```python
from build123d import *

# Parameters (mm, degrees)
SKETCH2_W           = 2.25
SKETCH2_H           = 25
BOSS_EXTRUDE1_DEPTH = 4
SKETCH4_OUTSIDE_W   = 76.3
SKETCH4_OUTSIDE_H   = 75.213
SKETCH4_OUTSIDE_R   = 3.514702834
CUT_EXTRUDE1_DEPTH  = 30
CUT_EXTRUDE1_TAPER  = 45


with BuildPart() as part:
    # Sketch2 → Revolve1 (revolve)
    with BuildSketch(Plane.XY):
        with Locations((1.125, 12.5)):
            Rectangle(SKETCH2_W, SKETCH2_H)
    revolve(axis=Axis((2.25, 25, 0), (0, -1, 0)))

    # Sketch3 → Boss-Extrude1 (add)
    with BuildSketch(Plane.XZ):
        Polygon((6.308429255, 0.02726243), (4.279214628, 3.541965265), (0.220785372, 3.541965265), (-1.808429255, 0.02726243), (0.220785372, -3.487440404), (4.279214628, -3.487440404), align=None)
    extrude(amount=BOSS_EXTRUDE1_DEPTH)

    # Sketch4 outside → Cut-Extrude1 (cut, through all)
    with BuildSketch(Plane(origin=(0, -4, 0), x_dir=(-1, 0, 0), z_dir=(0, -1, 0))):
        with Locations((-2.25, -0.0275)):
            Rectangle(SKETCH4_OUTSIDE_W, SKETCH4_OUTSIDE_H)
        with Locations((-2.25, -0.02726243)):
            Circle(SKETCH4_OUTSIDE_R, mode=Mode.SUBTRACT)
    extrude(amount=-CUT_EXTRUDE1_DEPTH, taper=CUT_EXTRUDE1_TAPER, mode=Mode.SUBTRACT)


solid = part.part
```
The model under review builds one solid part; all positions refer to its coordinate system, in mm. A direction names the side the tool comes from. Round coordinates to 2 decimals unless told otherwise and drop trailing zeros. Write each loop counter-clockwise with the first axis right and the second up, starting at its lowest first coordinate (ties: lowest second). Pieces come first, ordered by that corner, then holes.
(1) Mouldability with a two-part tool opening along X and no side actions: class faces 3 (the conical face through (0.434, -3.868, -3.135)), 4 (the flat face through (2, 25, 0)), 5 (the conical face through (4.081, -3.868, -3.127)) as +X half, -X half, draft (parallel to the pull), parting line (faces both ways), or undercut.
(2) We need section A-A on y = -1.25. Give the boundary of the cut face in (x, z), and give its area (3 significant figures).
(3) Insertion check: pin 1 (2 mm diameter, centred on x = 4, y = 1.5, fed in from +Z). The pin has a flat end and moves straight along its axis. Give the tip position at first contact, or say it passes through.
(4) Machinability: for faces 1 (the cylindrical face through (2.54, 12.68, -2.23)), 2 (the flat face through (-0.808, -1.972, -1.705)), which of the approach directions +Z, -Z, +X, -X, +Y, -Y give a long, thin tool a straight path to every point of the face, cutting with its end or side? Answer none if there is none.
(5) We need section B-B on y = 3.25. Give the boundary of the cut face in (x, z), and give its area (3 significant figures).
(6) Wall thickness on L1, parallel to Y at x = 0, z = 0.75; L2, parallel to Z at x = 2.25, y = 12.75; L3, parallel to X at y = 12.5, z = 1.5: over which ranges is each line inside the solid? List them lowest first.
Findings below:
1. face 3: -X half
1. face 4: draft
1. face 5: +X half
2. outline: (-1.81, 0.03) - (0.22, -3.49) - (4.28, -3.49) - (6.31, 0.03) - (4.28, 3.54) - (0.22, 3.54) - close
2. area: 42.8 mm2
3. pin 1: stops at z = 2.12
4. face 1: +Y
4. face 2: -Z, -X, +Y, -Y
5. outline: circle Ø4.5 at (2.25, 0)
5. area: 15.9 mm2
6. L1: y = -4 to 0
6. L2: z = -2.25 to 2.25
6. L3: x = 0.57 to 3.93
